Read the model definition and answer for the solid it produces. Units are mm, in the model's axes. Face numbers are marked on the shaded views. Coordinates: 2 decimals unless noted, no trailing zeros. Write each loop counter-clockwise with the first axis right and the second up, starting at its lowest first coordinate (ties: lowest second). Pieces come first, ordered by that corner, then holes. Notation, with made-up numbers: (66, 76) -> (125, 76) arc R20 ccw to (125, 82) -> close; hole circle Ø8 at (72.25, 84.5). An arc over 180 degrees is marked (long way). Return JSON: item names as keys, results as strings.
from build123d import *

# Parameters (mm, degrees)
SKETCH_R        = 40
SKETCH_R_2      = 13.2
PAD_DEPTH       = 2
SKETCH001_R     = 40
SKETCH001_R_2   = 36.5
PAD001_DEPTH    = 20
SKETCH002_W     = 2
SKETCH002_H     = 26.167402
SKETCH002_H_2   = 24.922537
SKETCH002_H_3   = 27.566788
POCKET_DEPTH    = 40.001
CHAMFER_SIZE    = 1
CHAMFER001_SIZE = 1
CHAMFER002_SIZE = 1


with BuildPart() as part:
    # Sketch → Pad (new body)
    with BuildSketch(Plane.XY):
        Circle(SKETCH_R)
        Circle(SKETCH_R_2, mode=Mode.SUBTRACT)
    extrude(amount=PAD_DEPTH)

    # Sketch001 (on Face4 of Pad) → Pad001 (join)
    with BuildSketch(Plane.XY.offset(2)):
        Circle(SKETCH001_R)
        Circle(SKETCH001_R_2, mode=Mode.SUBTRACT)
    extrude(amount=PAD001_DEPTH)

    # Sketch002 → Pocket (cut, through all)
    with BuildSketch(Plane.YZ):
        with Locations((5, 15.083701)):
            Rectangle(SKETCH002_W, SKETCH002_H)
        with Locations((-5, 14.461268)):
            Rectangle(SKETCH002_W, SKETCH002_H_2)
        with Locations((-15, 15.783394)):
            Rectangle(SKETCH002_W, SKETCH002_H_3)
    extrude(amount=-POCKET_DEPTH, mode=Mode.SUBTRACT)

    # Chamfer
    chamfer_edges = [part.edges().sort_by_distance(p)[0] for p in [
        (3.008522, 39.8867, 22),
    ]]
    chamfer(chamfer_edges, length=CHAMFER_SIZE)

    # Chamfer001
    chamfer001_edges = [part.edges().sort_by_distance(p)[0] for p in [
        (-40, 0, 22),
    ]]
    chamfer(chamfer001_edges, length=CHAMFER001_SIZE)

    # Chamfer002
    chamfer002_edges = [part.edges().sort_by_distance(p)[0] for p in [
        (-38.715902, -10.053803, 22),
    ]]
    chamfer(chamfer002_edges, length=CHAMFER002_SIZE)


solid = part.part
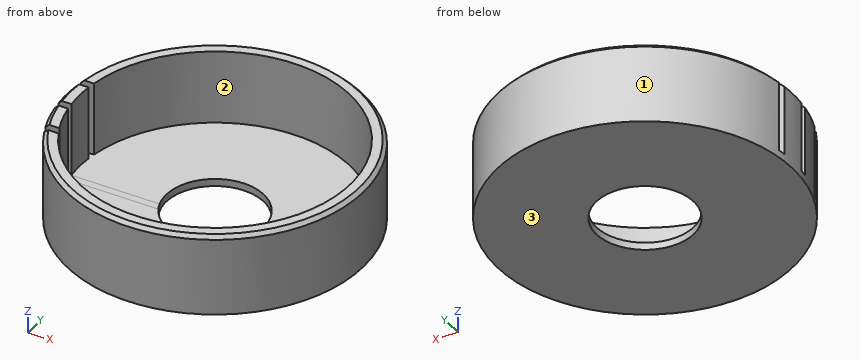
1. The part is cut by section B-B (z = 10). Determine the outline of the cut face in (x, y).
Taken from the geometry:
{"outline": "(-39.8, -4) -> (-36.28, -4) arc R36.5 cw to (-36.28, 4) -> (-39.8, 4) arc R40 ccw to start; (-39.55, -6) arc R40 ccw to (-37.47, -14) -> (-33.71, -14) arc R36.5 cw to (-36, -6) -> close; (-39.55, 6) -> (-36, 6) arc R36.5 cw (long way) to (-32.81, -16) -> (-36.66, -16) arc R40 ccw (long way) to start"}
2. Flat-ended cylindrical pins translate along their axes: pin 1 Ø1.5 at (x, y) = (20.5, -1) entering from +Z; pin 2 Ø5 at (x, z) = (-28, 10.5) entering from -Y; pin 3 Ø3 at (x, z) = (-34.5, 13.5) entering from +Y; pin 4 Ø8 at (x, y) = (2.5, -6.5) entering from +Z. Find the tip coordinate at first contact, or state that the pin passes through.
Taken from the geometry:
{"pin 1": "stops at z = 2", "pin 2": "stops at y = -30.82", "pin 3": "stops at y = 22.61", "pin 4": "passes through"}
3. For a pull along X with two mould halves and no side action, classify the marked faces 1, 2 and 3 as +X half, -X half, draft (parallel to the pull), parting line (faces both ways), or undercut.
Taken from the geometry:
{"face 1": "parting line", "face 2": "undercut", "face 3": "draft"}
4. The part is cut by section A-A (y = 0). Determine the outline of the cut face in (x, z), then the cut area to 3 significant figures.
Taken from the geometry:
{"outline": "(-40, 0) -> (-13.2, 0) -> (-13.2, 2) -> (-36.5, 2) -> (-36.5, 22) -> (-39, 22) -> (-40, 21) -> close; (13.2, 0) -> (40, 0) -> (40, 21) -> (39, 22) -> (36.5, 22) -> (36.5, 2) -> (13.2, 2) -> close", "area": "246 mm2"}
5. Consider L1, parallel to Y at x = 0, z = 17.25; L2, parallel to Y at x = 0, z = 1.3. Determine where each line is inside the solid, lowest interval first.
Taken from the geometry:
{"L1": "y = -40 to -36.5, 36.5 to 40", "L2": "y = -40 to -13.2, 13.2 to 40"}
